from build123d import *

# Parameters (mm, degrees)
RESSALTO_EXTRUS_O1_DEPTH          = 80
CORTE_EXTRUS_O2_REACH             = 103.336
ESBO_O2_W                         = 30
ESBO_O2_H                         = 30
CORTE_EXTRUS_O2_DIRECTION_2_DEPTH = 102.336074524
CORTE_EXTRUS_O3_REACH             = 103.336


with BuildPart() as part:
    # Esboço1 → Ressalto-extrusão1 (new body)
    with BuildSketch(Plane(origin=(0, 0, 0), x_dir=(0, 0, -1), z_dir=(1, 0, 0))):
        Polygon((-50, 7), (-24.019237886, 22), (-8.660254038, 22), (0, 37), (0, 0), (-18, 0), (-18, -8), (-43, -8), (-50, 1), align=None)
    extrude(amount=-RESSALTO_EXTRUS_O1_DEPTH)

    # Esboço2 → Corte-extrusão2 (cut, up to next)
    with BuildSketch(Plane.XY, mode=Mode.PRIVATE) as corte_extrus_o2_sk1:
        with Locations((-65, 22)):
            Rectangle(ESBO_O2_W, ESBO_O2_H)
    corte_extrus_o2_tool1 = extrude(corte_extrus_o2_sk1.sketch, amount=CORTE_EXTRUS_O2_REACH, mode=Mode.PRIVATE) & part.part
    add(corte_extrus_o2_tool1.solids().sort_by_distance((-65, 22, 0))[0], mode=Mode.SUBTRACT)

    # Esboço2 → Corte-extrusão2 direction 2 (cut)
    with BuildSketch(Plane.XY):
        with Locations((-65, 22)):
            Rectangle(ESBO_O2_W, ESBO_O2_H)
    extrude(amount=-CORTE_EXTRUS_O2_DIRECTION_2_DEPTH, mode=Mode.SUBTRACT)

    # Esboço3 → Corte-extrusão3 (cut, up to next)
    with BuildSketch(Plane.XY, mode=Mode.PRIVATE) as corte_extrus_o3_sk1:
        Polygon((-25, 37), (0, -8), (0, 37), align=None)
    corte_extrus_o3_tool1 = extrude(corte_extrus_o3_sk1.sketch, amount=CORTE_EXTRUS_O3_REACH, mode=Mode.PRIVATE) & part.part
    add(corte_extrus_o3_tool1.solids().sort_by_distance((-8.333333, 22, 0))[0], mode=Mode.SUBTRACT)


solid = part.part
The model under review builds one solid part; all positions refer to its coordinate system, in mm. A direction names the side the tool comes from. Give positions to 0.01 mm unless a question says otherwise; leave off trailing zeros. Loops run counter-clockwise (first coordinate to the right, second up) from the corner with the lowest first, then second, coordinate; pieces in that order, holes last. Notation, with made-up numbers: (83.25, -1.5) -> (129.25, -1.5) arc R25 ccw to (129.25, 12.5) -> close; hole circle Ø3 at (10.5, -27). An arc over 180 degrees is marked (long way). Answer as a JSON object with one key per item and string values. Group by question number.
Q1. Tool access review of faces 1 (the flat face through (-50, 15, 19)), 2 (the flat face through (-33, 22, 16)), 3 (the flat face through (-33, 15, 0)), 4 (the flat face through (-42, 0, 9)): name each direction out of +Z, -Z, +X, -X, +Y, -Y from which nothing blocks a thin tool from reaching the whole face with its end or side.
Q2. Take a section at B-B (z = 12.5). Write out the cut boundary in (x, y), plus the area to 3 significant figures.
Q3. Take a section at C-C (y = 20.5). Write out the cut boundary in (x, z), plus the area to 3 significant figures.
Q4. Insertion check: pin 1 (1 mm diameter, centred on y = 12, z = 8, fed in from +X); pin 2 (12 mm diameter, centred on x = -71, z = 39, fed in from +Y); pin 3 (8 mm diameter, centred on x = -46, y = 29, fed in from +Z). Each pin has a flat end and moves straight along its axis. Give the tip position at first contact, or say it passes through.
Q5. Wall thickness on line 1 along X through (y, z) = (22, 7); line 2 along Y through (x, z) = (-21, 19); line 3 along Y through (x, z) = (-53, 14): over which ranges is each line inside the solid? List them lowest first.
Q6. Take a section at A-A (x = -6). Write out the cut boundary in (y, z).
Q7. Take a section at D-D (x = -42.5). Write out the cut boundary in (y, z), plus the area to 3 significant figures.
Answer below:
{
 "1": {"face 1": "+Z, -Z, -X, +Y", "face 2": "+Z, +X, -X, +Y", "face 3": "-Z, +X, -X, +Y, -Y", "face 4": "-Z, +X, -X, -Y"},
 "2": {"outline": "(-80, 0) -> (-4.44, 0) -> (-16.67, 22) -> (-50, 22) -> (-50, 7) -> (-80, 7) -> close", "area": "1,080 mm2"},
 "3": {"outline": "(-50, 0) -> (-15.83, 0) -> (-15.83, 26.62) -> (-50, 26.62) -> close", "area": "909 mm2"},
 "4": {"pin 1": "stops at x = -10.83", "pin 2": "stops at y = 7", "pin 3": "stops at z = 6.93"},
 "5": {"line 1": "x = -50 to -16.67", "line 2": "y = -8 to 22", "line 3": "y = 0 to 7"},
 "6": {"outline": "(-8, 18) -> (0, 18) -> (0, 0) -> (2.8, 0) -> (2.8, 50) -> (1, 50) -> (-8, 43) -> close"},
 "7": {"outline": "(-8, 18) -> (0, 18) -> (0, 0) -> (37, 0) -> (22, 8.66) -> (22, 24.02) -> (7, 50) -> (1, 50) -> (-8, 43) -> close", "area": "1,190 mm2"}
}
